Job drawing, mm, ordinate dimensions from the low corner. One solid piece. A direction names the side the tool comes from. Give positions to 0.01 mm unless a question says otherwise; leave off trailing zeros. Write each loop counter-clockwise with the first axis right and the second up, starting at its lowest first coordinate (ties: lowest second). Pieces come first, ordered by that corner, then holes. Notation, with made-up numbers: (8, -16.75) - (19, -16.75) arc R12 ccw to (19, -2.75) - close; hole circle Ø5 at (-14.75, 81.25). An arc over 180 degrees is marked (long way). Use a Markdown table: item, result. Add a question column.
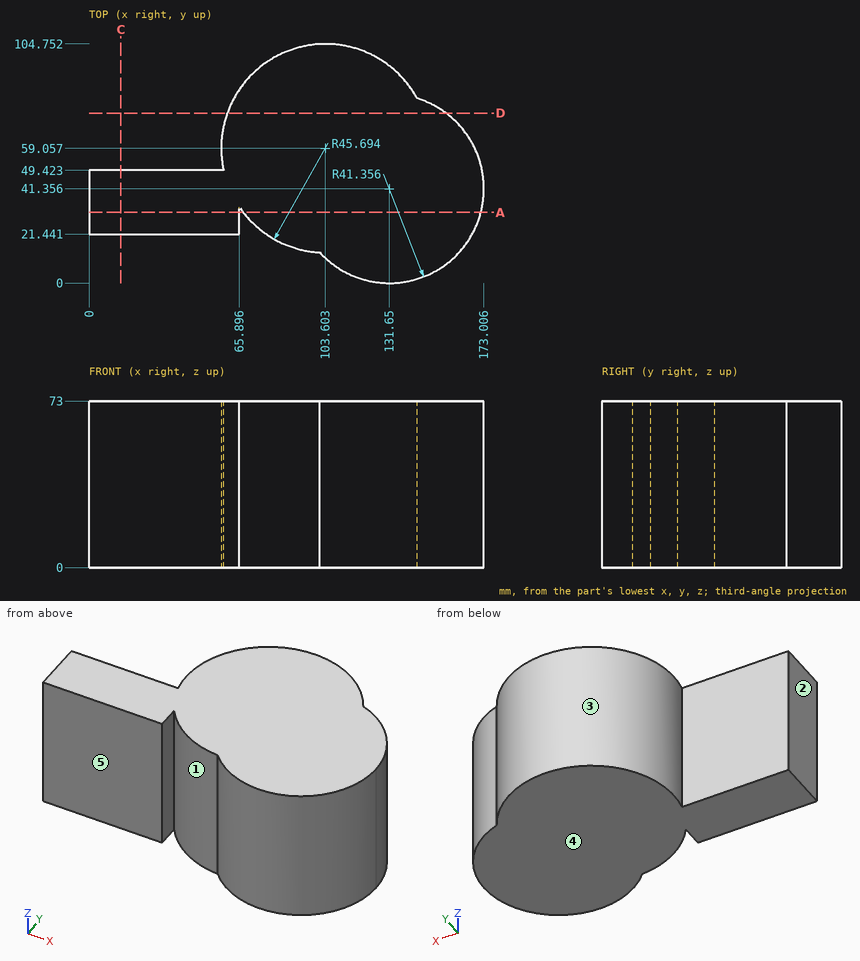
(1) Two-plate mould, pull along X, no slides. Class the marked faces 1, 2 and 3: +X half, -X half, draft (parallel to the pull), parting line (faces both ways), or undercut.
(2) Probe probe 1 along Y at (x, z) = (50, 30); probe 2 along X at (y, z) = (53, 14.5); probe 3 along Y at (x, z) = (152.5, 10.5). List the from-to ranges inside material, lowest first. Write a range as [from, to].
(3) Band-saw the part on A-A (y = 31). Write the cut outline in (x, z).
(4) Band-saw the part on C-C (x = 14). Write the cut outline in (y, z), then the cut area to 3 significant figures.
(5) Band-saw the part on D-D (y = 74.5). Write the cut outline in (x, z) (1 decimal), then the cut area to 3 significant figures.
(6) Which spindle directions (+Z, -Z, +X, -X, +Y, -Y) get a long thin tool onto all of the face, cutting with end or side? Do the marked faces 4 and 5. Say none if no direction does.
(7) Flat gauge pins, fed straight in: pin 1 (17.5 mm diameter, centred on x = 29, z = 52.5, fed in from +Y); pin 2 (13 mm diameter, centred on y = 27.5, z = 37, fed in from +X); pin 3 (3 mm diameter, centred on y = 82.5, z = 14, fed in from -X). Where does each tip first touch, or does it go through?
Model answer:
| question | item | result |
|---|---|---|
| 1 | face 1 | undercut |
| 1 | face 2 | -X half |
| 1 | face 3 | parting line |
| 2 | probe 1 | y = [21.44, 49.42] |
| 2 | probe 2 | x = [58.31, 171.33] |
| 2 | probe 3 | y = [5.64, 77.07] |
| 3 | outline | (0, 0) - (65.9, 0) - (65.9, 73) - (0, 73) - close; (67.54, 0) - (171.69, 0) - (171.69, 73) - (67.54, 73) - close |
| 4 | outline | (21.44, 0) - (49.42, 0) - (49.42, 73) - (21.44, 73) - close |
| 4 | area | 2,040 mm^2 |
| 5 | outline | (60.6, 0) - (156.4, 0) - (156.4, 73) - (60.6, 73) - close |
| 5 | area | 6,990 mm^2 |
| 6 | face 4 | -Z, +X, -X, +Y, -Y |
| 6 | face 5 | +Z, -Z, -X, -Y |
| 7 | pin 1 | stops at y = 49.42 |
| 7 | pin 2 | stops at x = 172.35 |
| 7 | pin 3 | stops at x = 63.52 |
